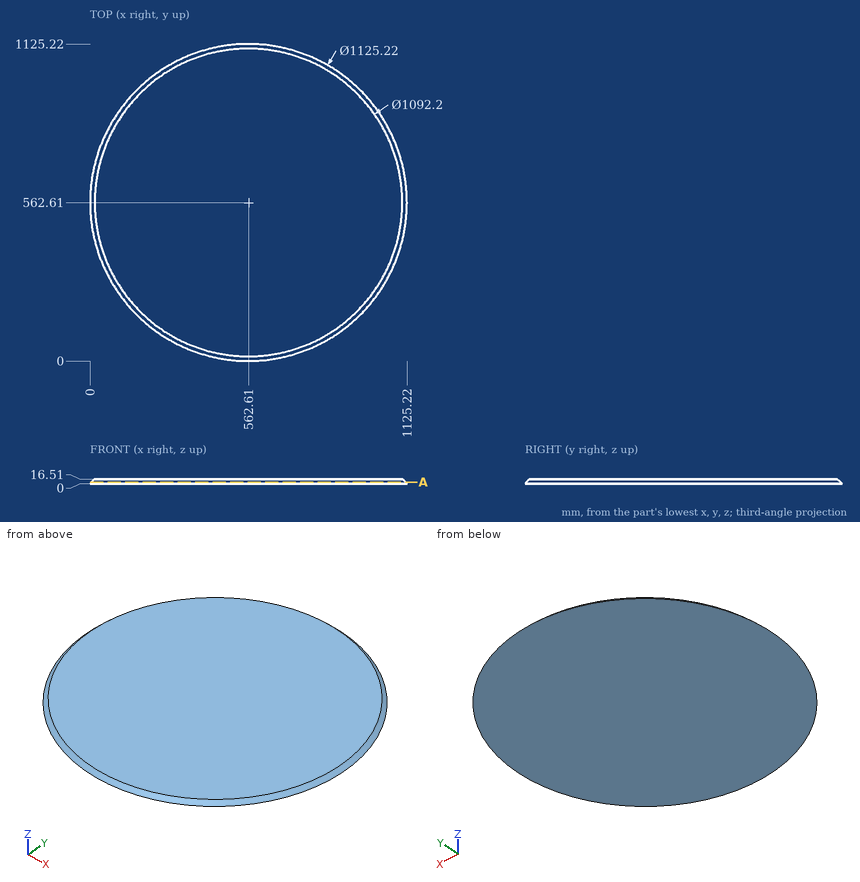
Answer from the drawing. Dimensions are ordinates in mm from the lowest x, y and z of the part. Round coordinates to 2 decimals unless told otherwise and drop trailing zeros. Write each loop counter-clockwise with the first axis right and the second up, starting at its lowest first coordinate (ties: lowest second). Pieces come first, ordered by that corner, then holes. Notation, with made-up numbers: (22.5, 50.5) - (62.5, 50.5) arc R16 ccw to (62.5, 77.5) - close; hole circle Ø1 at (82.25, 27.5). An arc over 180 degrees is marked (long way). One line per item, written item: value.
Q1. Each of these flat-tipped pins is pushed along its axis until it touches: P1, Ø1.5, axis at y = 877.5, z = 4, coming from the -X side; P2, Ø1.5, axis at x = 164, z = 11.5, coming from the +Y side; P3, Ø2, axis at x = 369, z = 9.5, coming from the +Y side. Where does it stop, or does it pass through?
The answers:
P1: stops at x = 100.17
P2: stops at y = 944.52
P3: stops at y = 1081.86
Q2. Find section A-A (z = 5.5). Determine the outline of the cut face in (x, y).
The answers:
outline: circle Ø1114.22 at (562.61, 562.61)
Q3. Straight lines are drawn through the part: line 1 (X direction, y = 840.5, z = 8); line 2 (X direction, y = 373, z = 8.25); line 3 (Y direction, x = 346, z = 10). For each, find the intervals that lie inside material, in ascending order. Write a range as from..to.
The answers:
line 1: x = 82.64..1042.58
line 2: x = 41.68..1083.54
line 3: y = 54.22..1071
